For this review, take the finished solid that the model builds, in its own axes (mm). Face numbers are marked on the shaded views. A direction names the side the tool comes from. Round coordinates to 2 decimals unless told otherwise and drop trailing zeros. Loops run counter-clockwise (first coordinate to the right, second up) from the corner with the lowest first, then second, coordinate; pieces in that order, holes last.
1) Take a section at A-A (x = -5). State the section outline as (y, z) points.
2) Wall thickness on L1, parallel to X at y = -0.8, z = -5; L2, parallel to Y at x = -19, z = -9; L3, parallel to Z at x = -11.75, y = -10.25: over which ranges is each line inside the solid? List them lowest first.
3) Insertion check: pin 1 (3 mm diameter, centred on x = -7.5, z = -9.5, fed in from -Y); pin 2 (4 mm diameter, centred on x = -14.5, y = -8.5, fed in from +Z); pin 3 (5 mm diameter, centred on x = -16, z = -5.5, fed in from -Y). Each pin has a flat end and moves straight along its axis. Give the tip position at first contact, or say it passes through.
4) Mouldability with a two-part tool opening along X and no side actions: class the marked faces 1, 2 and 3 as pulls with the +X half, pulls with the -X half, needs draft (parallel to the pull), parting line crosses it, or undercut.
5) Take a section at D-D (y = -6.5). State the section outline as (x, z) points.
6) Tool access review of the marked faces 4 and 5: name each direction out of +Z, -Z, +X, -X, +Y, -Y from which nothing blocks a thin tool from reaching the whole face with its end or side.
7) Take a section at C-C (y = -0.75). State the section outline as (x, z) points.
8) Take a section at B-B (x = -13). State the section outline as (y, z) points, then the cut area to 3 significant figures.
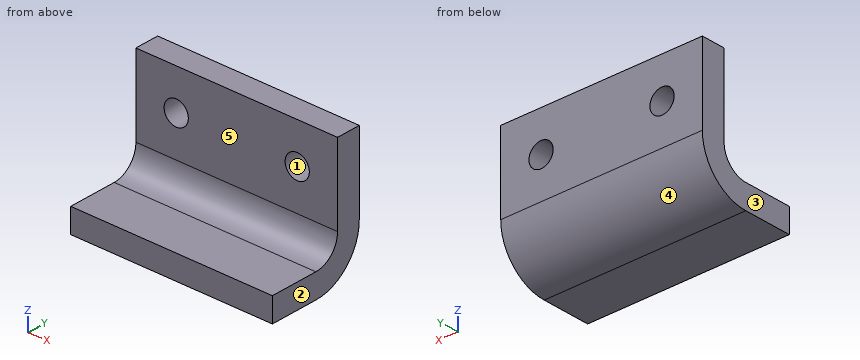
```python
from build123d import *

# Parameters (mm, degrees)
SKETCH1_W                = 25
SKETCH1_H                = 10
BASE_FLANGE1_DEPTH       = 3
F_3_0_3_DIAMETER_HOLE1_D = 3
SM_EDGE_FLANGE_1_DEPTH   = 25


# Sheet-metal steps are written as plain solids
with BuildPart() as part:
    # Sketch1 → Base-Flange1 (new body)
    with BuildSketch(Plane(origin=(0, 0, 0), x_dir=(1, 0, 0), z_dir=(0, 1, 0))):
        with Locations((-12.5, 5)):
            Rectangle(SKETCH1_W, SKETCH1_H)
    extrude(amount=-BASE_FLANGE1_DEPTH)

    # Ø3.0 (3) Diameter Hole1 (through all)
    with Locations(Plane(origin=(0, 0, 0), x_dir=(1, 0, 0), z_dir=(0, 1, 0))):
        with Locations((-20, 5), (-5, 5)):
            Hole(F_3_0_3_DIAMETER_HOLE1_D / 2)

    # 邊線-凸緣1 section (across the edge) → 邊線-凸緣1 (add)
    with BuildSketch(Plane(origin=(-25, -3, -13), x_dir=(0, 0, 1), z_dir=(1, 0, 0))):
        with BuildLine():
            Line((-3, 3), (-3, 9))
            Line((-3, 9), (0, 9))
            Line((0, 9), (0, 3))
            ThreePointArc((0, 3), (0.878679656, 0.878679656), (3, 0))
            Line((3, 0), (3, -3))
            ThreePointArc((3, -3), (-1.242640687, -1.242640687), (-3, 3))
        make_face()
    extrude(amount=SM_EDGE_FLANGE_1_DEPTH)


solid = part.part
```
Response:
1. outline: (-12, -16) - (-6, -16) arc R6 ccw to (0, -10) - (0, -6.5) - (-3, -6.5) - (-3, -10) arc R3 cw to (-6, -13) - (-12, -13) - close; (-3, -3.5) - (0, -3.5) - (0, 0) - (-3, 0) - close
2. L1: x = -25 to -21.5, -18.5 to -6.5, -3.5 to 0
2. L2: y = -3 to 0
2. L3: z = -16 to -13
3. pin 1: stops at y = -3.17
3. pin 2: stops at z = -13
3. pin 3: stops at y = -3
4. face 1: undercut
4. face 2: pulls with the +X half
4. face 3: pulls with the -X half
5. outline: (-25, -16) - (0, -16) - (0, -13) - (-25, -13) - close
6. face 4: -Z, +X, -X, +Y
6. face 5: +Z, +X, -X, -Y
7. outline: (-25, -12.9) - (0, -12.9) - (0, 0) - (-25, 0) - close; hole circle Ø3 at (-20, -5); hole circle Ø3 at (-5, -5)
8. outline: (-12, -16) - (-6, -16) arc R6 ccw to (0, -10) - (0, 0) - (-3, 0) - (-3, -10) arc R3 cw to (-6, -13) - (-12, -13) - close
8. area: 69.2 mm2
